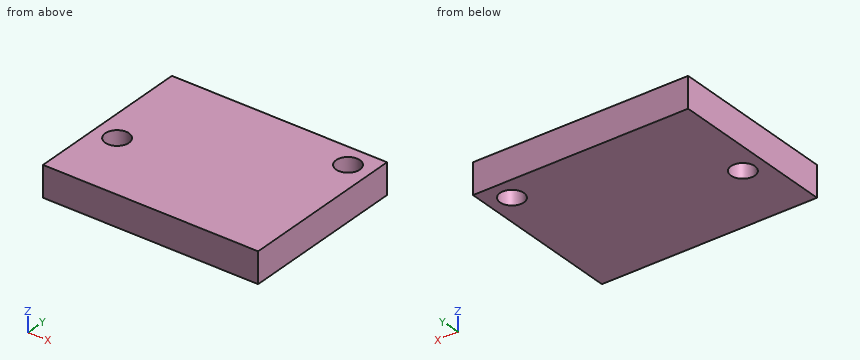
Autodesk Inventor part; units mm, degrees
ref_plane "YZ Plane" through (0, 0, 0) normal (1, 0, 0) x (0, 1, 0)
ref_plane "XZ Plane" through (0, 0, 0) normal (0, 1, 0) x (-1, 0, 0)
ref_plane "XY Plane" through (0, 0, 0) normal (0, 0, 1) x (1, 0, 0)
sketch "Sketch1" plane through (0, 0, 0) normal (0, 0, 1) x (1, 0, 0)
  line L0 (-14, 0) -> (14, 0)
  line L1 (14, 0) -> (14, 16)
  line L2 (14, 16) -> (-14, 16)
  line L3 (-14, 16) -> (-14, 0)
  circle A0 centre (-11.1, 2.85) radius 1.55
  circle A1 centre (11.1, 13.15) radius 1.55
  line L4 (-11.1, 2.85) -> (-14, 2.85) construction
  line L5 (11.1, 13.15) -> (14, 13.15) construction
  line L6 (11.1, 13.15) -> (11.1, 16) construction
  line L7 (-11.1, 2.85) -> (-11.1, 0) construction
  line L8 (-14, 0) -> (14, 0) construction
  line L9 (14, 0) -> (14, -6)
  line L10 (14, -6) -> (-14, -6)
  line L11 (-14, -6) -> (-14, 0)
  point P0 (0, 0)
  point P1 (0, 0)
  point P2 (14, 0)
  dimension "d0" = 3.1
  dimension "d1" = 22.2
  dimension "d2" = 10.3
  dimension "d3" = 16
  dimension "d4" = 28
  dimension "d5" = 22
extrude "Extrusion1" add sketch "Sketch1" along normal blind 4
properties part number "SwitchHolder_V1" material "Wood (Oak)"
CAD build for the part. Positions are in the model's coordinates, mm. Round coordinates to 2 decimals unless told otherwise and drop trailing zeros. Order: outer loops, then holes, each group sorted by start corner. A loop starts at its lowest first (then second) coordinate and runs counter-clockwise, first axis right, second up. Notation, with made-up numbers: (-37.5, -11.5) - (3.5, -11.5) arc R17 cw to (3.5, 2.5) - close; hole circle Ø6 at (55.5, 31). An arc over 180 degrees is marked (long way). Answer in a Markdown table with one row per item. Add a question column.
(1) Band-saw the part on A-A on y = 13.15. List the corners of the cut face in (x, z).
(2) Band-saw the part on C-C on z = 0.5. List the corners of the cut face in (x, y).
(3) Probe L1, parallel to Y at x = 11.1, z = 3.1; L2, parallel to Y at x = -11.1, z = 2.1; L3, parallel to X at y = 3.5, z = 2.75. List the from-to ranges inside material, lowest first. Write a range as [from, to].
(4) Band-saw the part on B-B on x = 11.1. List the corners of the cut face in (y, z), and give its area (3 significant figures).
Data:
| question | item | result |
|---|---|---|
| 1 | outline | (-14, 0) - (9.55, 0) - (9.55, 4) - (-14, 4) - close; (12.65, 0) - (14, 0) - (14, 4) - (12.65, 4) - close |
| 2 | outline | (-14, -6) - (14, -6) - (14, 16) - (-14, 16) - close; hole circle Ø3.1 at (-11.1, 2.85); hole circle Ø3.1 at (11.1, 13.15) |
| 3 | L1 | y = [-6, 11.6], [14.7, 16] |
| 3 | L2 | y = [-6, 1.3], [4.4, 16] |
| 3 | L3 | x = [-14, -12.51], [-9.69, 14] |
| 4 | outline | (-6, 0) - (11.6, 0) - (11.6, 4) - (-6, 4) - close; (14.7, 0) - (16, 0) - (16, 4) - (14.7, 4) - close |
| 4 | area | 75.6 mm^2 |
